Autodesk Inventor part; units mm, degrees
ref_plane "YZ Plane" through (0, 0, 0) normal (1, 0, 0) x (0, 1, 0)
ref_plane "XZ Plane" through (0, 0, 0) normal (0, 1, 0) x (-1, 0, 0)
ref_plane "XY Plane" through (0, 0, 0) normal (0, 0, 1) x (1, 0, 0)
sketch "Sketch1" plane through (0, 0, 0) normal (0, 0, 1) x (1, 0, 0)
  line L0 (-56.9976, 63.5) -> (0, 63.5)
  line L1 (0, 63.5) -> (-7.493, 63.5)
  line L2 (-7.493, 63.5) -> (-7.493, 57.15)
  line L3 (-56.9976, 63.5) -> (-49.5046, 63.5)
  line L4 (-49.5046, 63.5) -> (-49.5046, 57.15)
  line L5 (-56.9976, 63.5) -> (-56.9976, 0)
  line L6 (-56.9976, 0) -> (0, 0)
  line L7 (0, 0) -> (0, 63.5)
  line L8 (-28.4988, 0) -> (-28.4988, 11.1125)
  circle A0 centre (-28.4988, 11.1125) radius 4.7625
  dimension "d3" = 7.493
  dimension "d4" = 6.35
  dimension "d5" = 7.493
  dimension "d19" = 6.35
  dimension "d60" = 63.5
  dimension "d61" = 11.1125
  dimension "d62" = 9.525
extrude "Plate6" add sketch "Sketch1" along normal blind 3.175
sketch "Sketch6" plane through (0, 0, 0) normal (0, 0, -1) x (-1, 0, 0)
  line L0 (56.9976, 63.5) -> (56.9976, 0)
  line L1 (28.4988, 11.1125) -> (27.3076, 11.1125)
  line L2 (28.4988, 11.1125) -> (29.6894, 11.1125)
  circle A0 centre (28.4988, 11.1125) radius 4.7625
  circle A1 centre (28.4988, 11.1125) radius 4.7625
  line L3 (27.3076, 11.1125) -> (29.6888, 11.1125)
  line L4 (29.6888, 11.1125) -> (29.6888, 15.7239)
  line L5 (29.6888, 15.7239) -> (27.3076, 15.7239)
  line L6 (27.3076, 15.7239) -> (27.3076, 11.1125)
  line L7 (27.3076, 15.7239) -> (27.3076, 16.9145)
  line L8 (27.3076, 16.9145) -> (29.6888, 16.9145)
  line L9 (29.6888, 16.9145) -> (29.6888, 15.7239)
  point P0 (27.2012, 15.6948)
  point P1 (30.5454, 15.4129)
  dimension "d82" = 1.1906
  dimension "d86" = 2.3813
  dimension "d87" = 1.1906
extrude "Cut1" cut sketch "Sketch6" against normal blind 3.175 contours L7 L8 L9 A0 | A0 L5
sketch "Sketch7" plane through (-56.9976, 0, 0) normal (-1, 0, 0) x (0, 0, 1)
  line L0 (3.175, 0) -> (3.175, 63.5)
  line L1 (0, 63.5) -> (3.175, 63.5)
  line L2 (0, 63.5) -> (0, 0)
  line L3 (0, 0) -> (3.175, 0)
extrude "Extrusion2" add sketch "Sketch7" along normal blind 52.1462
sketch "Sketch8" plane through (0, 0, 3.175) normal (0, 0, 1) x (1, 0, 0)
  line L0 (0, 0) -> (-109.1438, 0)
  line L1 (-109.1438, 0) -> (-109.1438, 63.5)
  line L2 (-109.1438, 63.5) -> (-109.1438, 34.925)
  line L3 (-109.1438, 34.925) -> (-56.9976, 34.925)
  line L4 (-56.9976, 34.925) -> (-56.9976, 0)
  circle A0 centre (-75.5412, 57.15) radius 3.3782
  circle A1 centre (-75.5412, 41.275) radius 3.3782
  dimension "d71" = 28.575
  dimension "d72" = 52.1462
sketch "Sketch9" plane through (0, 0, 0) normal (0, 0, -1) x (-1, 0, 0)
  circle A0 centre (49.4976, 57.2287) radius 3.3
  circle A1 centre (7.4976, 57.2287) radius 3.3
extrude "Cut3" cut sketch "Sketch9" against normal blind 3.175
extrude "Cut4" cut sketch "Sketch8" against normal blind 3.175 contours L0 L1 L3 L4
sketch "Sketch10" plane through (0, 0, 3.175) normal (0, 0, 1) x (1, 0, 0)
  circle A0 centre (-90.6002, 57.15) radius 3.3782
  circle A1 centre (-90.6002, 41.275) radius 3.3782
extrude "Cut5" cut sketch "Sketch10" against normal blind 3.175
fillet "Fillet1" radius 25.4 2 edges at (-56.9976, 0, 1.5875) (0, 0, 1.5875)
sketch "Sketch11" plane through (0, 0, 3.175) normal (0, 0, 1) x (1, 0, 0)
  circle A0 centre (-90.6002, 57.15) radius 3.3782
  circle A1 centre (-90.6002, 41.275) radius 3.3782
  arc A2 (-25.4, 0) -> (0, 25.4) centre (-25.4, 25.4) ccw
  line L0 (0, 63.5) -> (0, 25.4)
  line L1 (-109.1438, 63.5) -> (0, 63.5)
  line L2 (-109.1438, 34.925) -> (-109.1438, 63.5)
  line L3 (-109.1438, 34.925) -> (-56.9976, 34.925)
  line L4 (-56.9976, 34.925) -> (-56.9976, 25.4)
  arc A3 (-56.9976, 25.4) -> (-31.5976, 0) centre (-31.5976, 25.4) ccw
  line L5 (-25.4, 0) -> (-31.5976, 0)
  circle A4 centre (-49.4976, 57.2287) radius 3.3
  circle A5 centre (-7.4976, 57.2287) radius 3.3
  line L6 (-29.6888, 15.7239) -> (-29.6888, 16.9145)
  line L7 (-29.6888, 16.9145) -> (-27.3076, 16.9145)
  line L8 (-27.3076, 16.9145) -> (-27.3076, 15.7239)
  line L9 (-27.3076, 15.7239) -> (-27.3088, 15.7239)
  arc A6 (-29.6888, 15.7239) -> (-27.3088, 15.7239) centre (-28.4988, 11.1125) ccw
  point P0 (0, 0)
equation "\"d67\" = Thickness"
equation "\"d75\" = Thickness"
equation "\"d77\" = Thickness"
equation "\"d79\" = Thickness"
equation "\"BendRadius\" = Thickness"
equation "\"BendReliefWidth\" = Thickness"
equation "\"BendReliefDepth\" = 0.5 * Thickness"
equation "\"CornerReliefSize\" = 4 * Thickness"
equation "\"MinimumRemnant\" = 2 * Thickness"
equation "\"TransitionRadius\" = BendRadius"
equation "\"JacobiRadiusSize\" = BendRadius"
equation "\"GapSize\" = Thickness"
equation "\"d8\" = BendRadius"
equation "\"d56\" = BendRadius"
equation "\"d63\" = BendRadius"
properties part number "arm mout" material "Steel"
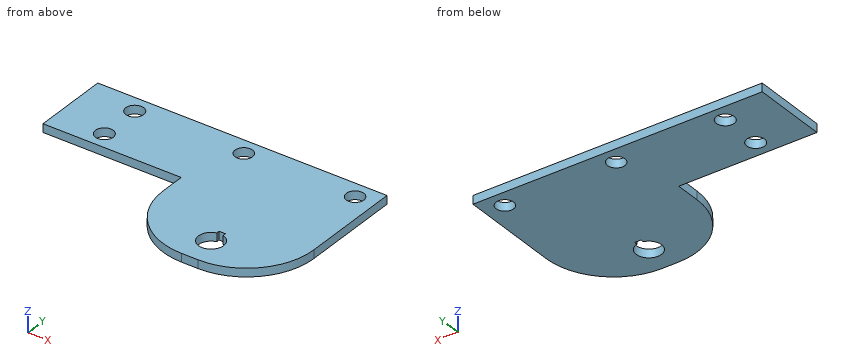
Source: CAD feature listing. Evaluate the final solid. Frame: model axes, mm. Coordinates: 2 decimals unless noted, no trailing zeros. Order: outer loops, then holes, each group sorted by start corner. A loop starts at its lowest first (then second) coordinate and runs counter-clockwise, first axis right, second up. Notation, with made-up numbers: (26, -32) - (62, -32) arc R17 ccw to (62, -21) - close; hole circle Ø9 at (-12, 40). An arc over 180 degrees is marked (long way). One line per item, written item: value.
1) Ray query, line 1 (Y direction, x = -92, z = 2.5) (3 decimals); line 2 (X direction, y = 29, z = 1.1); line 3 (Y direction, x = -72.5, z = 1.25) (3 decimals). Return the intervals inside material, ascending. Write a range as [from, to].
Computed values:
line 1: y = [34.925, 38.2], [44.35, 54.075], [60.225, 63.5]
line 2: x = [-57, 0]
line 3: y = [34.925, 63.5]
2) Contact query for flat-ended pins moving along their axis: pin 1 (6 mm diameter, centred on x = -49.5, y = 57.23, fed in from +Z); pin 2 (1.5 mm diameter, centred on x = -24, z = 0.5, fed in from -Y); pin 3 (1 mm diameter, centred on y = 16.5, z = 2, fed in from +X); pin 4 (1 mm diameter, centred on y = 16.5, z = 1, fed in from -X). Output: stop coordinate, or through.
Computed values:
pin 1: passes through
pin 2: stops at y = 0.01
pin 3: stops at x = -1.43
pin 4: stops at x = -55.57
3) Cut plane A-A on z = 2.4. State how many separate pieces and enclosed holes the cut face has, plus the area to 3 significant figures.
Computed values:
separate pieces: 1
enclosed holes: 5
area: 4,620 mm^2
4) Cut plane B-B on y = 27.5. Output: boundary loops of the cut face in (x, z) (3 decimals), plus the area to 3 significant figures.
Computed values:
outline: (-56.998, 0) - (0, 0) - (0, 3.175) - (-56.998, 3.175) - close
area: 181 mm^2
5) Cut plane C-C on x = -100.5. Output: boundary loops of the cut face in (y, z) (3 decimals).
Computed values:
outline: (34.925, 0) - (63.5, 0) - (63.5, 3.175) - (34.925, 3.175) - close
